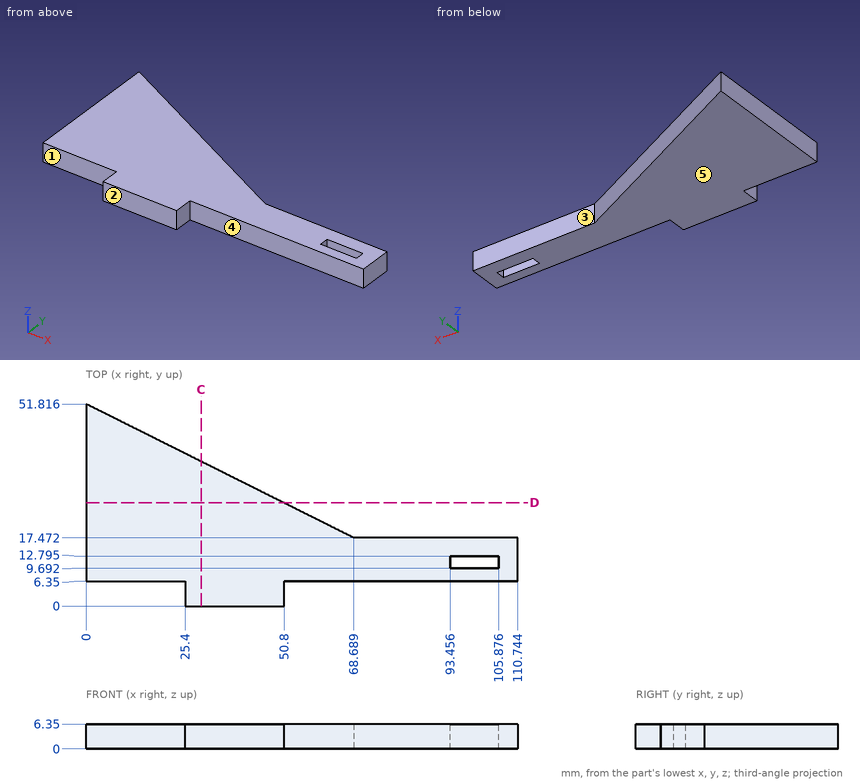
Geometry check sheet. Reference: drawing and pictorial views, mm from the part's lowest x, y, z. A direction names the side the tool comes from. Give positions to 0.01 mm unless a question says otherwise; leave off trailing zeros. Write each loop counter-clockwise with the first axis right and the second up, starting at its lowest first coordinate (ties: lowest second). Pieces come first, ordered by that corner, then holes. Notation, with made-up numbers: M 0,11.25 L 9,11.25 A21 ccw 9,48.25 Z; hole C 86,-17 d1. An arc over 180 degrees is marked long. Put each result on its own line as item: value. Start each with the question number.
1. Scan lines: line 1 along Y through (x, z) = (78, 0.75); line 2 along X through (y, z) = (3.5, 5); line 3 along Y through (x, z) = (31.5, 1.75) (1 decimal). Record each from-to range of solid material in increasing order. Write a range as [from, to].
2. Section check D-D (y = 26.5). Record the cut outline in (x, z).
3. Go/stop test with flat-tipped pins: pin 1 Ø3 at (x, z) = (7.5, 4) entering from -Y; pin 2 Ø8 at (x, y) = (33.5, 44) entering from +Z; pin 3 Ø3 at (x, z) = (84.5, 1.5) entering from +Y; pin 4 Ø1.9 at (y, z) = (3.5, 2) entering from -X. Record where each tip stops, or that it passes through.
4. Section check C-C (x = 29.5). Record the cut outline in (y, z).
5. Set-up check for the marked faces 1, 2, 3, 4 and 5: record each of +Z, -Z, +X, -X, +Y, -Y from which the full face is reachable in a straight line by a thin tool's end or side.
Answer list:
1. line 1: [6.35, 17.47]
1. line 2: [25.4, 50.8]
1. line 3: [0, 36.1]
2. outline: M 0,0 L 50.63,0 L 50.63,6.35 L 0,6.35 Z
3. pin 1: y = 6.35
3. pin 2: through
3. pin 3: y = 17.47
3. pin 4: x = 25.4
4. outline: M 0,0 L 37.07,0 L 37.07,6.35 L 0,6.35 Z
5. face 1: +Z, -Z, -X, -Y
5. face 2: +Z, -Z, +X, -X, -Y
5. face 3: +Z, -Z, +X, +Y
5. face 4: +Z, -Z, +X, -Y
5. face 5: -Z, +X, -X, +Y, -Y
